Input: part model. Units: mm. Frame: model coordinates. A direction names the side the tool comes from. Coordinates: 2 decimals unless noted, no trailing zeros. Order: outer loops, then holes, each group sorted by start corner. A loop starts at its lowest first (then second) coordinate and runs counter-clockwise, first axis right, second up. Notation, with made-up numbers: (12.25, -3.75) - (52.25, -3.75) arc R24 cw to (52.25, 9.25) - close; hole circle Ø5 at (-11, -23.75). An arc over 180 degrees is marked (long way). Use a Markdown table: item, result. Add a question column.
from build123d import *

# Parameters (mm, degrees)
SKETCH1_W           = 15
SKETCH1_H           = 25
SKETCH1_R           = 1.25
SKETCH1_W_2         = 10
SKETCH1_H_2         = 15
BOSS_EXTRUDE1_DEPTH = 5
SKETCH2_R           = 1.4
CUT_EXTRUDE1_DEPTH  = 4
FILLET1_R           = 5
FILLET2_R           = 1


with BuildPart() as part:
    # Sketch1 → Boss-Extrude1 (new body)
    with BuildSketch(Plane.XY):
        with Locations((7.5, -12.5)):
            Rectangle(SKETCH1_W, SKETCH1_H)
        with Locations((7.5, -3.75)):
            Circle(SKETCH1_R, mode=Mode.SUBTRACT)
        with Locations((7.5, -13.5)):
            Rectangle(SKETCH1_W_2, SKETCH1_H_2, mode=Mode.SUBTRACT)
    extrude(amount=BOSS_EXTRUDE1_DEPTH)

    # Sketch2 → Cut-Extrude1 (cut)
    with BuildSketch(Plane.XZ.offset(25)):
        with Locations(Location((7.5, 2.5, 0), (0, 0, 270))):
            Circle(SKETCH2_R)
    extrude(amount=-CUT_EXTRUDE1_DEPTH, mode=Mode.SUBTRACT)

    # Fillet1
    fillet1_edges = [part.edges().sort_by_distance(p)[0] for p in [
        (0, 0, 2.5),
        (15, 0, 2.5),
        (15, -25, 2.5),
        (0, -25, 2.5),
    ]]
    fillet(fillet1_edges, radius=FILLET1_R)

    # Fillet2
    fillet2_edges = [part.edges().sort_by_distance(p)[0] for p in [
        (12.5, -21, 2.5),
        (12.5, -6, 2.5),
        (2.5, -6, 2.5),
        (2.5, -21, 2.5),
    ]]
    fillet(fillet2_edges, radius=FILLET2_R)


solid = part.part
1) Pull-direction query (Y, two-part tool) for faces 1 (the flat face through (2, -12, 0)), 2 (the cylindrical face through (13, -24, 3)), 3 (the cylindrical face through (12.199, -20.715, 2.535)); classes: pulls with the +Y half, pulls with the -Y half, needs draft (parallel to the pull), parting line crosses it, or undercut.
2) Cut plane B-B (x = 7.5). Return the cut outline in (y, z), and give its area (3 significant figures).
3) Material intervals for L1, parallel to Y at x = 7.5, z = 3.1; L2, parallel to Y at x = 7, z = 4.55; L3, parallel to X at y = -16.25, z = 2.9, sorted ascending.
4) Cut plane A-A (y = -16). Return the cut outline in (x, z), and give its area (3 significant figures).
5) Reachability of faces 4 (the flat face through (15, -13, 2)), 5 (the cylindrical face through (6.133, -23.028, 2.803)), 6 (the flat face through (12.5, -14, 2)) from +Z, -Z, +X, -X, +Y, -Y: full face, straight path, thin tool, end or side. Return the list, or none.
6) Contact query for flat-ended pins moving along their axis: P1, Ø2, axis at x = 7.5, y = -3.75, coming from the -Z side; P2, Ø3, axis at x = 13.5, z = 1, coming from the +Y side; P3, Ø2.5, axis at x = 7.5, z = 2.5, coming from the -Y side. Output: stop coordinate, or through.
7) Cut plane D-D (z = 2.5). Return the cut outline in (x, y), and give its area (3 significant figures).
8) Cut plane C-C (z = 0.55). Return the cut outline in (x, y).
Computed:
| question | item | result |
|---|---|---|
| 1 | face 1 | needs draft |
| 1 | face 2 | pulls with the -Y half |
| 1 | face 3 | undercut |
| 2 | outline | (-25, 0) - (-21, 0) - (-21, 1.1) - (-25, 1.1) - close; (-25, 3.9) - (-21, 3.9) - (-21, 5) - (-25, 5) - close; (-6, 0) - (-5, 0) - (-5, 5) - (-6, 5) - close; (-2.5, 0) - (0, 0) - (0, 5) - (-2.5, 5) - close |
| 2 | area | 26.3 mm2 |
| 3 | L1 | y = -6 to -5, -2.5 to 0 |
| 3 | L2 | y = -25 to -21, -6 to -4.9, -2.6 to 0 |
| 3 | L3 | x = 0 to 2.5, 12.5 to 15 |
| 4 | outline | (0, 0) - (2.5, 0) - (2.5, 5) - (0, 5) - close; (12.5, 0) - (15, 0) - (15, 5) - (12.5, 5) - close |
| 4 | area | 25.0 mm2 |
| 5 | face 4 | +Z, -Z, +X, +Y, -Y |
| 5 | face 5 | -Y |
| 5 | face 6 | +Z, -Z |
| 6 | P1 | passes through |
| 6 | P2 | stops at y = -0.42 |
| 6 | P3 | stops at y = -6 |
| 7 | outline | (0, -20) arc R5 ccw to (5, -25) - (6.1, -25) - (6.1, -21) - (3.5, -21) arc R1 cw to (2.5, -20) - (2.5, -7) arc R1 cw to (3.5, -6) - (11.5, -6) arc R1 cw to (12.5, -7) - (12.5, -20) arc R1 cw to (11.5, -21) - (8.9, -21) - (8.9, -25) - (10, -25) arc R5 ccw to (15, -20) - (15, -5) arc R5 ccw to (10, 0) - (5, 0) arc R5 ccw to (0, -5) - close; hole circle Ø2.5 at (7.5, -3.75) |
| 7 | area | 188 mm2 |
| 8 | outline | (0, -20) arc R5 ccw to (5, -25) - (10, -25) arc R5 ccw to (15, -20) - (15, -5) arc R5 ccw to (10, 0) - (5, 0) arc R5 ccw to (0, -5) - close; hole (2.5, -20) arc R1 ccw to (3.5, -21) - (11.5, -21) arc R1 ccw to (12.5, -20) - (12.5, -7) arc R1 ccw to (11.5, -6) - (3.5, -6) arc R1 ccw to (2.5, -7) - close; hole circle Ø2.5 at (7.5, -3.75) |
